Build history of the part. All positions in model axes, mm. Face numbers are marked on the shaded views. A direction names the side the tool comes from. Round coordinates to 2 decimals unless told otherwise and drop trailing zeros. Write each loop counter-clockwise with the first axis right and the second up, starting at its lowest first coordinate (ties: lowest second). Pieces come first, ordered by that corner, then holes. Notation, with made-up numbers: (54, -8.5) -> (112, -8.5) arc R35 ccw to (112, 30.5) -> close; hole circle Ø6 at (-13, 4.25). An arc over 180 degrees is marked (long way). Answer in a Markdown table with one row per item.
```python
from build123d import *

# Parameters (mm, degrees)
FILLET1_R       = 0.3556
HEX_2_DEPTH     = 2.286
THDSCHPAT_COUNT = 37
THDSCHPAT_PITCH = 0.772297297


with BuildPart() as part:
    # BodySke → Base-Revolve (revolve)
    with BuildSketch(Plane.XY):
        Polygon((0, 0), (0, 3.48615), (0.4826, 3.96875), (4.826, 3.96875), (4.826, 2.413), (67.85356, 2.413), (68.326, 1.94056), (68.326, 0), align=None)
    revolve(axis=Axis((-31.75, 0, 0), (1, 0, 0)))

    # Fillet1
    fillet1_edges = [part.edges().sort_by_distance(p)[0] for p in [
        (4.826, -2.413, 0),
    ]]
    fillet(fillet1_edges, radius=FILLET1_R)

    # Sketch2 → Hex-PreBroach (revolve, cut)
    with BuildSketch(Plane.XY):
        Polygon((0, 1.98501), (2.286, 1.98501), (3.432046058, 0), (0, 0), align=None)
    revolve(axis=Axis((0, 0, 0), (1, 0, 0)), mode=Mode.SUBTRACT)

    # Sketch3 → Hex 2 (cut)
    with BuildSketch(Plane(origin=(0, 0, 0), x_dir=(0, 0.5, 0.866025404), z_dir=(-1, 0, 0))):
        Polygon((1.146046058, 1.98501), (-1.146046058, 1.98501), (-2.292092116, 0), (-1.146046058, -1.98501), (1.146046058, -1.98501), (2.292092116, 0), align=None)
    extrude(amount=-HEX_2_DEPTH, mode=Mode.SUBTRACT)

    # ThdSchSke → ThreadSchematic (revolve, cut)
    with BuildSketch(Plane.XY):
        Polygon((39.751, -1.94056), (39.420193951, -2.413), (39.420193951, -3.01625), (40.081806049, -3.01625), (40.081806049, -2.413), align=None)
    threadschematic = revolve(axis=Axis((-3.175, 0, 0), (1, 0, 0)), mode=Mode.SUBTRACT)

    # ThdSchPat: ThreadSchematic ×37
    with Locations(*[(i * THDSCHPAT_PITCH, 0, 0) for i in range(1, THDSCHPAT_COUNT)]):
        add(threadschematic, mode=Mode.SUBTRACT)


solid = part.part
```
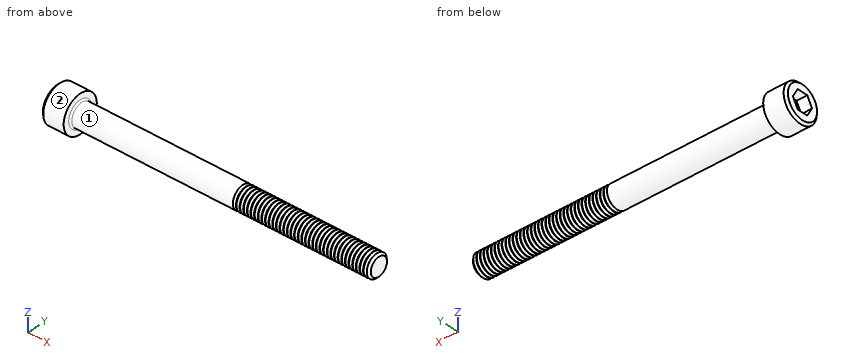
Q1. Drop flat-ended pins along their axis: P1, Ø3, axis at x = 8.5, z = -0.5, coming from the -Y side; P2, Ø3, axis at x = 20.5, y = 1.5, coming from the +Z side; P3, Ø2, axis at x = 12, y = -1, coming from the -Z side. Give the stop position or say it passes through.
A:
| item | result |
|---|---|
| P1 | y = -2.41 |
| P2 | z = 2.41 |
| P3 | z = -2.41 |
Q2. Saw through at A-A on x = 35.5. Write the cut outline in (y, z).
A:
| item | result |
|---|---|
| outline | circle Ø4.83 at (0, 0) |
Q3. Wall check: line 1 (X direction, y = 3, z = 1.25); line 2 (X direction, y = 1.5, z = 1); line 3 (Z direction, x = 35, y = -0.25). Give the ranges that are in metal, low to high. Write a range as [from, to].
A:
| item | result |
|---|---|
| line 1 | [0, 4.83] |
| line 2 | [2.39, 68.33] |
| line 3 | [-2.4, 2.4] |
Q4. Which spindle directions (+Z, -Z, +X, -X, +Y, -Y) get a long thin tool onto all of the face, cutting with end or side? Do the marked faces 1 and 2. Say none if no direction does.
A:
| item | result |
|---|---|
| face 1 | +X |
| face 2 | +X, -X |
